from build123d import *

# Parameters (mm, degrees)
CROQUIS1_R              = 1.5
SALIENTE_EXTRUIR1_DEPTH = 10
CROQUIS2_R              = 1.5
CROQUIS2_W              = 34
CROQUIS2_H              = 12.5
SALIENTE_EXTRUIR2_DEPTH = 6.25
CROQUIS3_W              = 25
CROQUIS3_H              = 5
CORTAR_EXTRUIR1_DEPTH   = 15
CROQUIS4_W              = 30
CROQUIS4_H              = 5
CORTAR_EXTRUIR2_DEPTH   = 30
CROQUIS6_W              = 40
CROQUIS6_H              = 7.662708713
CORTAR_EXTRUIR3_DEPTH   = 60
REDONDEO1_R             = 10


with BuildPart() as part:
    # Croquis1 → Saliente-Extruir1 (new body)
    with BuildSketch(Plane.XY):
        with BuildLine():
            Line((0, -5), (171.25, -5))
            ThreePointArc((171.25, -5), (176.25, 0), (171.25, 5))
            Line((171.25, 5), (85.625, 15))
            Line((85.625, 15), (0, 5))
            ThreePointArc((0, 5), (-5, 0), (0, -5))
        make_face()
        with Locations((171.25, 0)):
            Circle(CROQUIS1_R, mode=Mode.SUBTRACT)
        Circle(CROQUIS1_R, mode=Mode.SUBTRACT)
        with Locations((114.8954508, 0)):
            Circle(CROQUIS1_R, mode=Mode.SUBTRACT)
    extrude(amount=SALIENTE_EXTRUIR1_DEPTH)

    # Croquis2 → Saliente-Extruir2 (add, symmetric)
    # profile 1 of 2: a face of its own
    with BuildSketch(Plane.XY.offset(5)):
        with BuildLine():
            Line((171.25, 5), (161.25, 5))
            Line((161.25, 5), (161.25, -5))
            Line((161.25, -5), (171.25, -5))
            ThreePointArc((171.25, -5), (176.25, 0), (171.25, 5))
        make_face()
        with Locations((171.25, 0)):
            Circle(CROQUIS2_R, mode=Mode.SUBTRACT)
    # profile 2 of 2: a face of its own
    with BuildSketch(Plane.XY.offset(5)):
        with Locations((114.8954508, 1.25)):
            Rectangle(CROQUIS2_W, CROQUIS2_H)
        with Locations((114.8954508, 0)):
            Circle(CROQUIS2_R, mode=Mode.SUBTRACT)
    extrude(amount=SALIENTE_EXTRUIR2_DEPTH, both=True)

    # Croquis3 → Cortar-Extruir1 (cut)
    with BuildSketch(Plane.XZ.offset(5)):
        with Locations((176.25, 5)):
            Rectangle(CROQUIS3_W, CROQUIS3_H)
    extrude(amount=-CORTAR_EXTRUIR1_DEPTH, mode=Mode.SUBTRACT)

    # Croquis4 → Cortar-Extruir2 (cut)
    with BuildSketch(Plane.XZ.offset(5)):
        with Locations((112.94374, 5)):
            Rectangle(CROQUIS4_W, CROQUIS4_H)
    extrude(amount=-CORTAR_EXTRUIR2_DEPTH, mode=Mode.SUBTRACT)

    # Croquis6 → Cortar-Extruir3 (cut)
    with BuildSketch(Plane.XZ.offset(5)):
        with Locations((-5, 11.331354357)):
            Rectangle(CROQUIS6_W, CROQUIS6_H)
        with Locations((-5, -1.331354357)):
            Rectangle(CROQUIS6_W, CROQUIS6_H)
    extrude(amount=-CORTAR_EXTRUIR3_DEPTH, mode=Mode.SUBTRACT)

    # Redondeo1
    # the kernel refuses this fillet: 10 mm, written as the material it adds along each edge
    with BuildSketch(Plane(origin=(15, -5, 2.5), x_dir=(-1, 0, 0), z_dir=(0, 1, 0))) as redondeo1_piece_1_section:
        with BuildLine():
            CenterArc((6.614378278, -10), REDONDEO1_R, 90, 41.409622109)
            Line((0, -2.5), (-0.132287566, -2.35))
            ThreePointArc((-0.132287566, -2.35), (-0.2, -1.25), (-0.2, 0))
            Line((-0.2, 0), (0, 0.2))
            Line((0, 0.2), (6.614378278, 0.2))
            Line((6.614378278, 0.2), (6.614378278, 0))
        make_face()
    redondeo1_piece_1 = extrude(amount=28.287770512, mode=Mode.PRIVATE)
    redondeo1_piece_1 = split(redondeo1_piece_1, bisect_by=Plane(origin=(12.547080383, 6.465352453, 1.89633879), z_dir=(0.11599990937510621, -0.9932492240243469, 0)), keep=Keep.TOP, mode=Mode.PRIVATE)
    add(redondeo1_piece_1)
    with BuildSketch(Plane(origin=(15, -5, 7.5), x_dir=(0, 0, 1), z_dir=(0, 1, 0))) as redondeo1_piece_2_section:
        with BuildLine():
            CenterArc((10, -6.614378278), REDONDEO1_R, 138.590377891, 41.409622109)
            Line((0, -6.614378278), (-0.2, -6.614378278))
            Line((-0.2, -6.614378278), (-0.2, 0))
            Line((-0.2, 0), (0, 0.2))
            ThreePointArc((0, 0.2), (1.25, 0.2), (2.35, 0.132287566))
            Line((2.35, 0.132287566), (2.5, 0))
        make_face()
    redondeo1_piece_2 = extrude(amount=28.287770512, mode=Mode.PRIVATE)
    redondeo1_piece_2 = split(redondeo1_piece_2, bisect_by=Plane(origin=(12.547080383, 6.465352453, 8.10366121), z_dir=(0.11599990937510621, -0.9932492240243469, 0)), keep=Keep.TOP, mode=Mode.PRIVATE)
    add(redondeo1_piece_2)


solid = part.part
For this review, take the finished solid that the model builds, in its own axes (mm). A direction names the side the tool comes from. Round coordinates to 2 decimals unless told otherwise and drop trailing zeros. Write each loop counter-clockwise with the first axis right and the second up, starting at its lowest first coordinate (ties: lowest second). Pieces come first, ordered by that corner, then holes. Notation, with made-up numbers: (11.25, -20) - (70.25, -20) arc R19 cw to (70.25, 14) - close; hole circle Ø9 at (40, 33.25). An arc over 180 degrees is marked (long way). Use a Markdown table: item, result.
Q1. Clearance check with flat-ended pins moving along their axes: pin 1 (1.4 mm diameter, centred on y = -0.5, z = -0.5, fed in from -X); pin 2 (2.5 mm diameter, centred on y = 7, z = 6, fed in from +X); pin 3 (6 mm diameter, centred on x = 81.5, z = 6, fed in from +Y); pin 4 (2.5 mm diameter, centred on x = 171.25, y = 0, fed in from +Z). State where each tip first meets the part, or that it passes through.
Derived:
| item | result |
|---|---|
| pin 1 | stops at x = 14.77 |
| pin 2 | stops at x = 163.75 |
| pin 3 | stops at y = 14.87 |
| pin 4 | passes through |
Q2. We need section C-C (x = 64). Give the boundary of the cut face in (y, z).
Derived:
| item | result |
|---|---|
| outline | (-5, 0) - (12.47, 0) - (12.47, 10) - (-5, 10) - close |
Q3. The part is to be moulded in two halves that separate along Y. For faces 1 (the flat face through (129.04, 9.93, 4.93)), 2 (the cylindrical face through (11.874, 0.794, 1.872)), 3 (the cylindrical face through (113.4, 0.1, 0.6)), say which applies: pulls with the +Y half, pulls with the -Y half, needs draft (parallel to the pull), parting line crosses it, or undercut.
Derived:
| item | result |
|---|---|
| face 1 | pulls with the +Y half |
| face 2 | needs draft |
| face 3 | undercut |
Q4. Machinability: for faces 4 (the flat face through (127.944, 2, 5)), 5 (the flat face through (169, 0, -1.25)), 6 (the flat face through (169, 0, 7.5)), which of the approach directions +Z, -Z, +X, -X, +Y, -Y give a long, thin tool a straight path to every point of the face, cutting with its end or side? Answer none if there is none.
Derived:
| item | result |
|---|---|
| face 4 | +Y, -Y |
| face 5 | -Z, +X, -X, +Y, -Y |
| face 6 | +X, +Y, -Y |
Q5. We need section B-B (y = 0). State how many separate pieces and enclosed holes the cut face has, plus the area to 3 significant figures.
Derived:
| item | result |
|---|---|
| separate pieces | 5 |
| enclosed holes | 0 |
| area | 1,570 mm2 |
Q6. We need section A-A (z = 5.5). Give the boundary of the cut face in (x, y) (3 decimals).
Derived:
| item | result |
|---|---|
| outline | (0, -5) - (97.944, -5) - (97.944, 13.561) - (85.625, 15) - (0, 5) arc R5 ccw to start; (127.944, -5) - (163.75, -5) - (163.75, 5.876) - (127.944, 10.058) - close; hole circle Ø3 at (0, 0) |
Q7. We need section D-D (x = 140.5). Give the boundary of the cut face in (y, z).
Derived:
| item | result |
|---|---|
| outline | (-5, 0) - (8.59, 0) - (8.59, 10) - (-5, 10) - close |
Q8. Wall thickness on line 1 along X through (y, z) = (0, 6.1); line 2 along X through (y, z) = (0, -0.1); line 3 along Y through (x, z) = (0, 4.05): over which ranges is each line inside the solid? List them lowest first.
Derived:
| item | result |
|---|---|
| line 1 | x = -5 to -1.5, 1.5 to 97.94, 127.94 to 163.75 |
| line 2 | x = 97.9 to 113.4, 116.4 to 131.9, 161.25 to 169.75, 172.75 to 176.25 |
| line 3 | y = -5 to -1.5, 1.5 to 5 |
